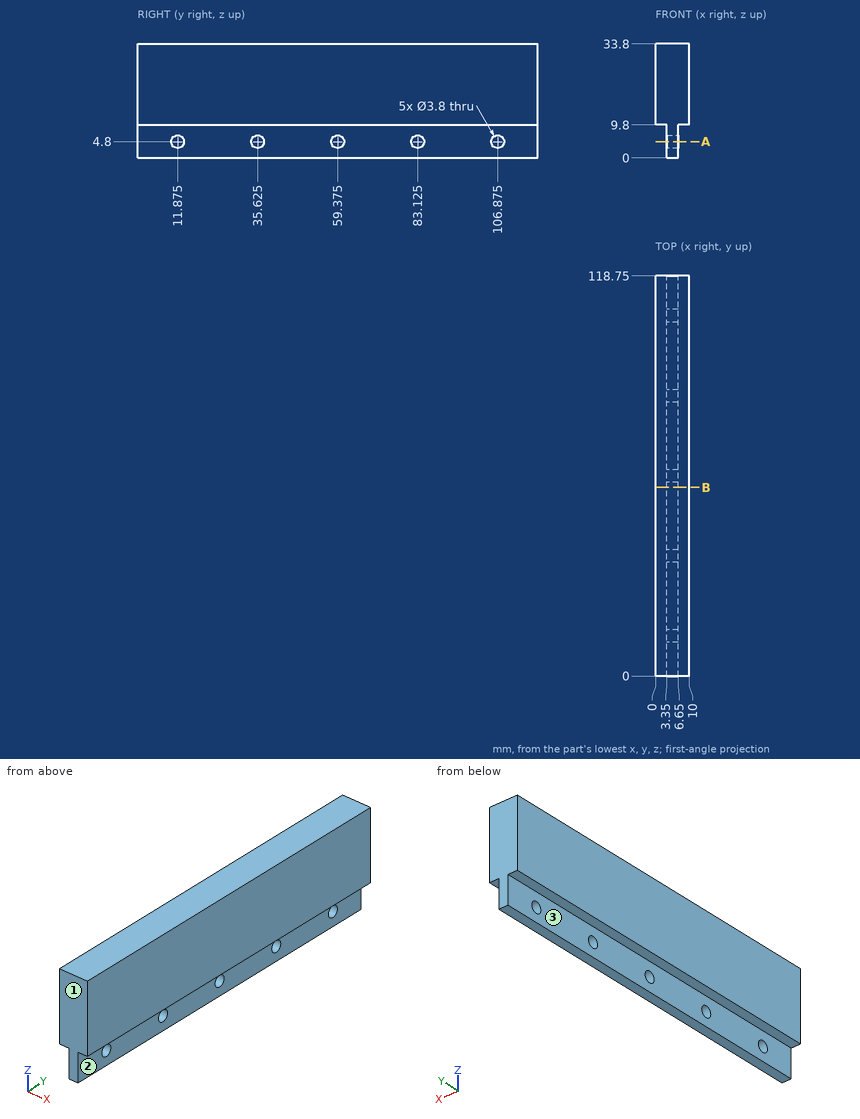
Verification items for this drawing (mm, ordinates from the low corner). A direction names the side the tool comes from. Give positions to 0.01 mm unless a question says otherwise; leave off trailing zeros. Write each loop counter-clockwise with the first axis right and the second up, starting at its lowest first coordinate (ties: lowest second). Pieces come first, ordered by that corner, then holes. Notation, with made-up numbers: (70.5, -33) - (126.5, -33) arc R27 ccw to (126.5, -11) - close; hole circle Ø2 at (5, 80.5). An arc over 180 degrees is marked (long way). Answer as CSV lines item,"result". Start each with the question number.
1. Sectioned sample at A-A (z = 4.8). Record the boundary of the cut face in (x, y) (3 decimals).
2. Thickness scan on line 1 (Y direction, x = 5, z = 4.8) (3 decimals); line 2 (Z direction, x = 7.75, y = 64.5); line 3 (X direction, y = 89, z = 5.5). Record the ranges inside material, lowest first.
3. Depth check by flat-ended pin: pin 1 (2.5 mm diameter, centred on y = 59.375, z = 4.8, fed in from -X); pin 2 (5 mm diameter, centred on y = 83.125, z = 4.8, fed in from +X); pin 3 (5 mm diameter, centred on y = 48.5, z = 4.5, fed in from -X); pin 4 (2.5 mm diameter, centred on x = 8.5, y = 41, fed in from -Z). Enter the tip coordinate at first touch or a pass-through.
4. Set-up check for the marked faces 1, 2 and 3: record each of +Z, -Z, +X, -X, +Y, -Y from which the full face is reachable in a straight line by a thin tool's end or side.
5. Sectioned sample at B-B (y = 56). Record the boundary of the cut face in (x, z), then the cut area to 3 significant figures.
Derived:
1,outline,"(3.35, 0) - (6.65, 0) - (6.65, 9.975) - (3.35, 9.975) - close; (3.35, 13.775) - (6.65, 13.775) - (6.65, 33.725) - (3.35, 33.725) - close; (3.35, 37.525) - (6.65, 37.525) - (6.65, 57.475) - (3.35, 57.475) - close; (3.35, 61.275) - (6.65, 61.275) - (6.65, 81.225) - (3.35, 81.225) - close; (3.35, 85.025) - (6.65, 85.025) - (6.65, 104.975) - (3.35, 104.975) - close; (3.35, 108.775) - (6.65, 108.775) - (6.65, 118.75) - (3.35, 118.75) - close"
2,line 1,"0 to 9.975, 13.775 to 33.725, 37.525 to 57.475, 61.275 to 81.225, 85.025 to 104.975, 108.775 to 118.75"
2,line 2,"9.8 to 33.8"
2,line 3,"3.35 to 6.65"
3,pin 1,"through"
3,pin 2,"x = 6.65"
3,pin 3,"x = 3.35"
3,pin 4,"z = 9.8"
4,face 1,"+Z, -Z, +X, -X, -Y"
4,face 2,"-Z, +X, +Y, -Y"
4,face 3,"-Z, -X, +Y, -Y"
5,outline,"(0, 9.8) - (3.35, 9.8) - (3.35, 0) - (6.65, 0) - (6.65, 9.8) - (10, 9.8) - (10, 33.8) - (0, 33.8) - close"
5,area,"272 mm²"
